Here's how the part is built. I have some questions about the finished solid (model axes, mm). Face numbers are marked on the shaded views. A direction names the side the tool comes from. Round coordinates to 2 decimals unless told otherwise and drop trailing zeros. Write each loop counter-clockwise with the first axis right and the second up, starting at its lowest first coordinate (ties: lowest second). Pieces come first, ordered by that corner, then holes. Notation, with made-up numbers: (32, -29) - (49, -29) arc R16 cw to (49, -20) - close; hole circle Ø1 at (29.5, -40). An arc over 180 degrees is marked (long way). One line per item, written item: value. Start each with the question number.
Item 1: Imagine slicing it at A-A, the plane y = -1.5. Please give me the cut outline in (x, z), then the cut area to 3 significant figures.
Item 2: Thinking about a two-plate mould opening in Z: for the marked faces 1, 2, 3 and 4, which applies, released by +Z, released by -Z, zero draft, split by the parting line, or undercut?
Item 3: Imagine slicing it at B-B, the plane x = 12. Please give me the cut outline in (y, z).
Item 4: For the marked faces 5 and 6, which set-ups out of +Z, -Z, +X, -X, +Y, -Y let a thin tool reach every point of the face, with its end or its side?
Item 5: If I drill on line 1 (X direction, y = -10, z = 1.5); line 2 (Z direction, x = 15.5, y = -5); line 3 (X direction, y = -1.25, z = -6), over which ranges is the centre line in solid material (lowest first)?
Item 6: For P1, Ø9, axis at x = -60.38, z = 0, coming from the -Y side; P2, Ø3, axis at x = -33.5, y = -11, coming from the -Z side; P3, Ø5, axis at y = -17.5, z = 14.5, coming from the +X side, each with a flat end and sliding along its axis, tell me the tip position at first contact or that it passes through.
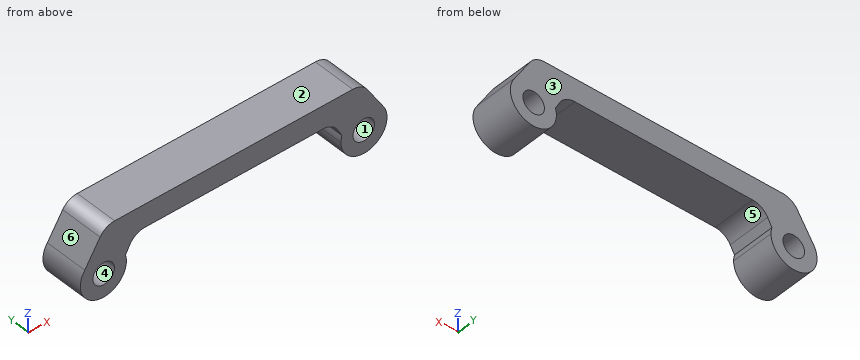
```python
from build123d import *

# Parameters (mm, degrees)
F1_DEPTH = 20
F3_D     = 10
F4_DEPTH = 20
F6_D     = 10


with BuildPart() as f1:
    # F0 (on Front) → F1 (new body)
    with BuildSketch(Plane.XZ):
        with BuildLine():
            ThreePointArc((-69.147074, 6.296465), (-63.81471, -10.168074), (-49.810232, 0))
            ThreePointArc((-49.810232, 0), (-49.915818, 1.499006), (-50.230489, 2.96841))
            ThreePointArc((-50.230489, 2.96841), (-58.650888, 10.531798), (-69.147074, 6.296465))
        make_face()
    extrude(amount=F1_DEPTH)

    # F3 (through all)
    with Locations(Plane.XZ.offset(20)):
        with Locations((-60.503781, 0)):
            Hole(F3_D / 2)

    # F0 (on Front) → F4 (join)
    with BuildSketch(Plane.XZ):
        with BuildLine():
            ThreePointArc((-69.147074, 6.296465), (-63.81471, -10.168074), (-49.810232, 0))
            ThreePointArc((-49.810232, 0), (-49.915818, 1.499006), (-50.230489, 2.96841))
            ThreePointArc((-50.230489, 2.96841), (-58.650888, 10.531798), (-69.147074, 6.296465))
        make_face()
        with BuildLine():
            ThreePointArc((-69.147074, 6.296465), (-58.650888, 10.531798), (-50.230489, 2.96841))
            Line((-50.230489, 2.96841), (-48.257435, 6.552011))
            ThreePointArc((-48.257435, 6.552011), (-45.319574, 9.580772), (-41.249421, 10.693549))
            Line((-41.249421, 10.693549), (0, 10.693549))
            Line((0, 10.693549), (0, 21.212202))
            Line((0, 21.212202), (-55.27229, 21.212202))
            ThreePointArc((-55.27229, 21.212202), (-59.123882, 20.223994), (-62.023932, 17.503511))
            Line((-62.023932, 17.503511), (-69.147074, 6.296465))
        make_face()
    extrude(amount=F4_DEPTH)

    # F6 (through all)
    with Locations(Plane(origin=(0, 0, 0), x_dir=(1, 0, 0), z_dir=(0, 1, 0))):
        with Locations((-60.377855, 0)):
            Hole(F6_D / 2)

    # F7: F1 across plane


with BuildPart() as f1_1:
    add(f1.part)
    add(f1.part.mirror(Plane.YZ))


solid = f1_1.part
```
Values follow:
1. outline: (-69.15, 6.3) arc R10.69 ccw (long way) to (-49.81, 0) arc R10.69 ccw to (-50.23, 2.97) - (-48.26, 6.55) arc R8 cw to (-41.25, 10.69) - (41.25, 10.69) arc R8 cw to (48.26, 6.55) - (50.23, 2.97) arc R10.69 ccw to (49.81, 0) arc R10.69 ccw (long way) to (69.15, 6.3) - (62.02, 17.5) arc R8 ccw to (55.27, 21.21) - (-55.27, 21.21) arc R8 ccw to (-62.02, 17.5) - close; hole circle Ø10 at (-60.38, 0); hole circle Ø10 at (60.38, 0)
1. area: 1,970 mm^2
2. face 1: undercut
2. face 2: released by +Z
2. face 3: zero draft
2. face 4: undercut
3. outline: (-20, 10.69) - (0, 10.69) - (0, 21.21) - (-20, 21.21) - close
4. face 5: -Z, +Y, -Y
4. face 6: +Z, -X, +Y, -Y
5. line 1: x = -71.09 to -65.15, -55.61 to -49.92, 49.92 to 55.61, 65.15 to 71.09
5. line 2: z = 10.69 to 21.21
5. line 3: x = -69.36 to -51.65, 51.65 to 69.36
6. P1: passes through
6. P2: stops at z = 10.69
6. P3: stops at x = 65.52
